```python
from build123d import *

# Parameters (mm, degrees)
SKETCH172_W     = 28
SKETCH172_H     = 105
PAD044_DEPTH    = 1.6
SKETCH173_R     = 1
POCKET023_DEPTH = 5
FILLET020_R     = 2


with BuildPart() as part:
    # Sketch172 (on DatumPlane) → Pad044 (new body)
    with BuildSketch(Plane(origin=(0, 19.5, -5), x_dir=(1, 0, 0), z_dir=(0, 0, 1))):
        with Locations((0, -40.5)):
            Rectangle(SKETCH172_W, SKETCH172_H)
    extrude(amount=PAD044_DEPTH)

    # Sketch173 → Pocket023 (cut)
    with BuildSketch(Plane.XY):
        with Locations((10, -13.5)):
            Circle(SKETCH173_R)
        with Locations((-6, 3.5)):
            Circle(SKETCH173_R)
    extrude(amount=-POCKET023_DEPTH, mode=Mode.SUBTRACT)

    # Fillet020
    fillet020_edges = [part.edges().sort_by_distance(p)[0] for p in [
        (14, 31.5, -4.2),
        (-14, 31.5, -4.2),
        (14, -73.5, -4.2),
        (-14, -73.5, -4.2),
    ]]
    fillet(fillet020_edges, radius=FILLET020_R)


solid = part.part
```
Here's how the part is built. I have some questions about the finished solid (model axes, mm). Coordinates: 2 decimals unless noted, no trailing zeros. Order: outer loops, then holes, each group sorted by start corner. A loop starts at its lowest first (then second) coordinate and runs counter-clockwise, first axis right, second up. Notation, with made-up numbers: (-29, 63.25) -> (-12, 63.25) arc R15 cw to (-12, 88.25) -> close; hole circle Ø10 at (76.5, 68). An arc over 180 degrees is marked (long way). Return JSON: item names as keys, results as strings.
1) If I drill on probe 1 along Y at (x, z) = (-6, -4.1); probe 2 along Y at (x, z) = (10, -3.8), over which ranges is the centre line in solid material (lowest first)?
Conclusion:
{"probe 1": "y = -73.5 to 2.5, 4.5 to 31.5", "probe 2": "y = -73.5 to -14.5, -12.5 to 31.5"}
2) If we section it at A-A on x = 10: List the corners of the cut face in (y, z) for me.
Conclusion:
{"outline": "(-73.5, -5) -> (-14.5, -5) -> (-14.5, -3.4) -> (-73.5, -3.4) -> close; (-12.5, -5) -> (31.5, -5) -> (31.5, -3.4) -> (-12.5, -3.4) -> close"}
3) If we section it at B-B on y = 3.5: List the corners of the cut face in (x, z) for me.
Conclusion:
{"outline": "(-14, -5) -> (-7, -5) -> (-7, -3.4) -> (-14, -3.4) -> close; (-5, -5) -> (14, -5) -> (14, -3.4) -> (-5, -3.4) -> close"}
4) Thinking about a two-plate mould opening in X: for faces 1 (the cylindrical face through (13.4, 30.93, -4.19)), 2 (the flat face through (0, -20, -5)), 3 (the cylindrical face through (9.783, -14.476, -4.189)), 4 (the cylindrical face through (-13.43, -72.9, -4.19)), which applies, +X half, -X half, draft (parallel to the pull), parting line (faces both ways), or undercut?
Conclusion:
{"face 1": "+X half", "face 2": "draft", "face 3": "undercut", "face 4": "-X half"}
